The model under review builds one solid part; all positions refer to its coordinate system, in mm. Face numbers are marked on the shaded views. Give positions to 0.01 mm unless a question says otherwise; leave off trailing zeros. Order: outer loops, then holes, each group sorted by start corner. A loop starts at its lowest first (then second) coordinate and runs counter-clockwise, first axis right, second up. Notation, with made-up numbers: (33, 6) -> (44, 6) arc R17 ccw to (44, 26) -> close; hole circle Ø7 at (-35.5, -16.5). An arc over 180 degrees is marked (long way). Use one line per item in the form item = value.
```python
from build123d import *

# Parameters (mm, degrees)
F1_DEPTH = 25.4
F2_R     = 12.7
F3_R     = 5.9718786186
F4_DEPTH = 25.401
F5_W     = 19.05
F5_H     = 62.6034842774
F6_DEPTH = 25.4


with BuildPart() as f1:
    # F0 (on Front) → F1 (new body)
    with BuildSketch(Plane.XZ):
        Polygon((0, 0), (43.3889701962, 0), (0, 49.6006347239), align=None)
    extrude(amount=F1_DEPTH)

    # F2
    f2_edges = [f1.edges().sort_by_distance(p)[0] for p in [
        (0, -12.7, 0),
    ]]
    fillet(f2_edges, radius=F2_R)

    # F3 (on face) → F4 (cut, through all)
    with BuildSketch(Plane.XZ.offset(25.4)):
        with Locations((12.7, 12.7)):
            Circle(F3_R)
    extrude(amount=-F4_DEPTH, mode=Mode.SUBTRACT)

    # F5 (on face) → F6 (cut)
    with BuildSketch(Plane(origin=(24.5799735671, 0, 21.5017357432), x_dir=(0, 1, 0), z_dir=(0.7526638098, 0, 0.6584050344))):
        with Locations((-12.1681662276, 4.3852257229)):
            Rectangle(F5_W, F5_H)
    extrude(amount=-F6_DEPTH, mode=Mode.SUBTRACT)


solid = f1.part
```
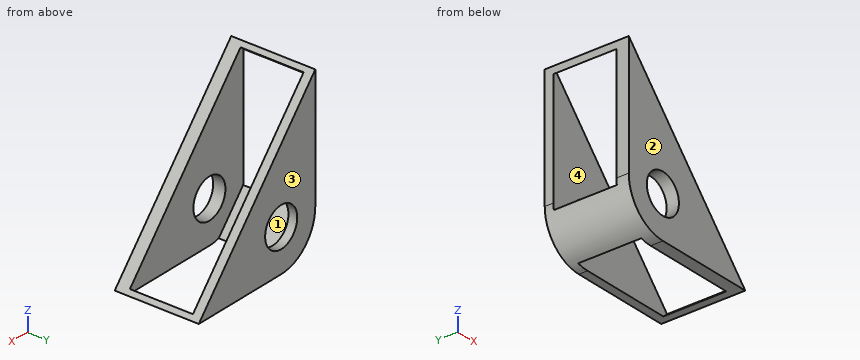
1. Add section D-D on x = 8.5. Give the boundary of the cut face in (y, z).
Values:
outline = (-25.4, 0.71) -> (0, 0.71) -> (0, 8.45) -> (-2.64, 8.45) -> (-2.64, 1.31) -> (-21.69, 1.31) -> (-21.69, 8.45) -> (-25.4, 8.45) -> close; (-25.4, 16.95) -> (-21.69, 16.95) -> (-21.69, 39.88) -> (-25.4, 39.88) -> close; (-2.64, 16.95) -> (0, 16.95) -> (0, 39.88) -> (-2.64, 39.88) -> close
2. For pin 1 Ø15.5 at (x, z) = (12.7, 12.7) entering from +Y; pin 2 Ø10 at (y, z) = (-5, 10.5) entering from +X, all flat-tipped, find the tip position at first contact; note any pin that passes through.
Values:
pin_1 = 0
pin_2 = 38.06
3. For L1, parallel to Y at x = 11, z = 6; L2, parallel to Z at x = 12.7, y = -1.4; L3, parallel to X at y = -2.25, z = 21.5, list the stretches that pass through material, from the lowest coordinate up.
Values:
L1 = -25.4 to -21.69, -2.64 to 0
L2 = 0 to 6.73, 18.67 to 35.08
L3 = 0 to 24.58
4. Add section B-B on x = 26. Give the boundary of the cut face in (y, z).
Values:
outline = (-25.4, 0) -> (-21.69, 0) -> (-21.69, 19.88) -> (-25.4, 19.88) -> close; (-2.64, 0) -> (0, 0) -> (0, 19.88) -> (-2.64, 19.88) -> close
5. Add section A-A on y = -9. Give the boundary of the cut face in (x, z).
Values:
outline = (0, 47.41) -> (1.08, 48.36) -> (0, 49.6) -> close; (0.13, 10.87) arc R12.7 ccw to (9.22, 0.49) -> close; (40.88, 0) -> (43.39, 0) -> (42.3, 1.24) -> close
6. The part is to be moulded in two halves that separate along Y. For the marked faces 1, 2, 3 and 4, say which applies: +Y half, -Y half, draft (parallel to the pull), parting line (faces both ways), or undercut.
Values:
face_1 = undercut
face_2 = -Y half
face_3 = +Y half
face_4 = undercut
7. Add section C-C on z = 36. Give the boundary of the cut face in (x, y).
Values:
outline = (0, -25.4) -> (11.9, -25.4) -> (11.9, -21.69) -> (0, -21.69) -> close; (0, -2.64) -> (11.9, -2.64) -> (11.9, 0) -> (0, 0) -> close
